The figure shows three views and two pictorial views of one solid part (mm, origin at its lowest corner). Answer the questions. Coordinates: 2 decimals unless noted, no trailing zeros. Order: outer loops, then holes, each group sorted by start corner. A loop starts at its lowest first (then second) coordinate and runs counter-clockwise, first axis right, second up. Notation, with made-up numbers: M 7.25,-25 L 14.25,-25 A27 cw 14.25,-4 Z; hole C 44,35.5 d10. An arc over 180 degrees is marked long. Answer in a Markdown table with one row per item. Add a question column.
Item 1: The part is cut by section B-B (z = 0.15). Write down the section's boundary in (x, y), then the cut area to 3 significant figures.
Item 2: The part is cut by section A-A (x = 20.5). Write down the section's boundary in (y, z).
Item 3: The part is cut by section C-C (x = 26.25). Write down the section's boundary in (y, z).
Item 4: Consider line 1 (Y direction, x = 19.5, z = 0.25); line 2 (X direction, y = 15, z = 0.3); line 3 (X direction, y = 14.75, z = 0.25). Determine where each line is inside the solid, lowest interval first. Write a range as from..to.
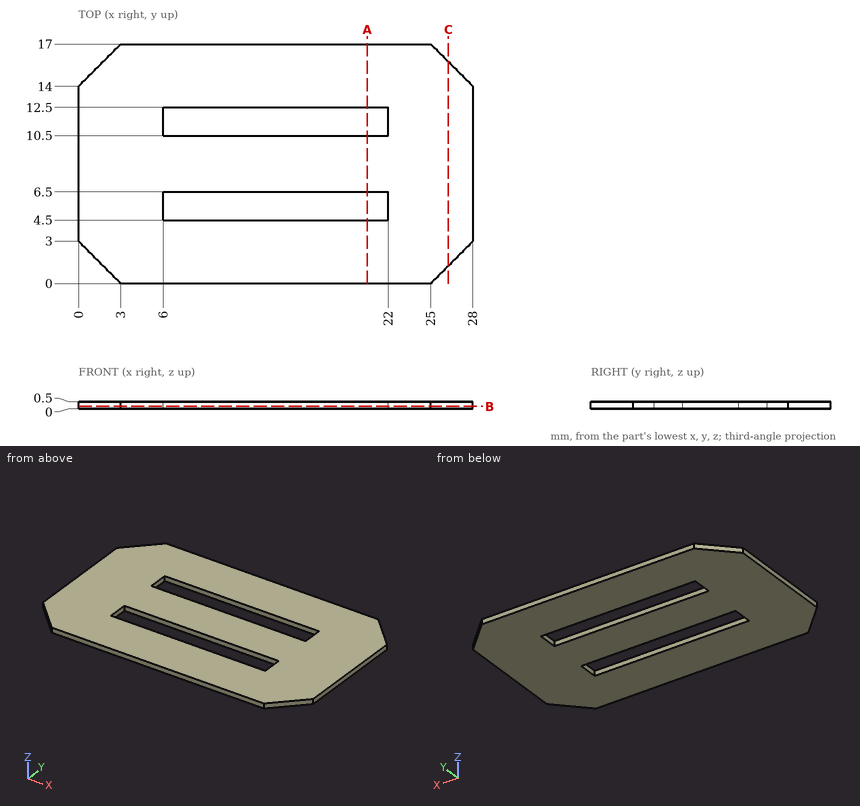
Reply:
| question | item | result |
|---|---|---|
| 1 | outline | M 0,3 L 3,0 L 25,0 L 28,3 L 28,14 L 25,17 L 3,17 L 0,14 Z; hole M 6,4.5 L 22,4.5 L 22,6.5 L 6,6.5 Z; hole M 6,10.5 L 22,10.5 L 22,12.5 L 6,12.5 Z |
| 1 | area | 394 mm2 |
| 2 | outline | M 0,0 L 4.5,0 L 4.5,0.5 L 0,0.5 Z; M 6.5,0 L 10.5,0 L 10.5,0.5 L 6.5,0.5 Z; M 12.5,0 L 17,0 L 17,0.5 L 12.5,0.5 Z |
| 3 | outline | M 1.25,0 L 15.75,0 L 15.75,0.5 L 1.25,0.5 Z |
| 4 | line 1 | y = 0..4.5, 6.5..10.5, 12.5..17 |
| 4 | line 2 | x = 1..27 |
| 4 | line 3 | x = 0.75..27.25 |
